The model under review builds one solid part; all positions refer to its coordinate system, in mm. Give positions to 0.01 mm unless a question says otherwise; leave off trailing zeros. Loops run counter-clockwise (first coordinate to the right, second up) from the corner with the lowest first, then second, coordinate; pieces in that order, holes last. Notation, with made-up numbers: M 22,-31 L 53,-31 A20 ccw 53,-21 Z; hole C 74,81.25 d3. An arc over 180 degrees is marked long. Return JSON: item names as keys, results as strings. Group by question number.
```python
from build123d import *
from build123d import SkipClean  # not in build123d's __all__

# Parameters (mm, degrees)
F1_DEPTH = 6


with BuildPart() as f1:
    # F0 (on Front) → F1 (new body)
    with BuildSketch(Plane.XZ):
        with BuildLine():
            ThreePointArc((-2.5981308411, 69.4027374984), (-23.7554424043, 60.1122052703), (-34.4088510941, 39.607310612))
            Line((-34.4088510941, 39.607310612), (-40, 0))
            Line((-40, 0), (0, 0))
            Line((0, 0), (0, 8))
            ThreePointArc((0, 8), (-26.7312756631, 33.7492995345), (-2, 61.4251288657))
            Line((-2, 61.4251288657), (-2.5981308411, 69.4027374984))
        make_face()
    extrude(amount=F1_DEPTH)

    # F2: F1 across plane


with BuildPart() as f1_1:
    add(f1.part, clean=False)
    with SkipClean():  # cleaning this boolean's faces spoils the solid; the shape is the same uncleaned
        add(f1.part.mirror(Plane.YZ), clean=False)


solid = f1_1.part
```
(1) Add section D-D (z = 7). Write out the cut boundary in (x, y).
(2) For pin 1 (1.5 mm diameter, centred on x = -4, y = -1.5, fed in from +Z); pin 2 (1.5 mm diameter, centred on x = 21.5, y = -1, fed in from +Z); pin 3 (1 mm diameter, centred on y = -4.5, z = 21.5, fed in from +X), all flat-tipped, find the tip position at first contact; note any pin that passes through.
(3) Add section A-A (x = -5.5). Write out the cut boundary in (y, z).
(4) For probe 1 along X at (y, z) = (-2, 15.5); probe 2 along Z at (x, y) = (21.5, -3.85); probe 3 along X at (y, z) = (-3.7, 58), list the stretches that pass through material, from the lowest coordinate up.
(5) Mouldability with a two-part tool opening along X and no side actions: class faces 1 (the flat face through (37.165, -2.958, 20.081)), 2 (the flat face through (2.3, -3, 65.4)), 3 (the flat face through (1, -3, 0)), 4 (the flat face through (-2.3, -3, 65.4)) as released by +X, released by -X, zero draft, split by the parting line, or undercut.
(6) Add section C-C (y = -5.15). Write out the cut boundary in (x, z).
(7) Add section B-B (z = 18). Write out the cut boundary in (x, y), and give its area (3 significant figures).
Verdict:
{
 "1": {"outline": "M -39.01,-6 L 39.01,-6 L 39.01,0 L -39.01,0 Z"},
 "2": {"pin 1": "stops at z = 69.35", "pin 2": "stops at z = 62.62", "pin 3": "stops at x = 37.04"},
 "3": {"outline": "M -6,0 L 0,0 L 0,8.57 L -6,8.57 Z; M -6,60.93 L 0,60.93 L 0,69.06 L -6,69.06 Z"},
 "4": {"probe 1": "x = -37.81 to -18.57, 18.57 to 37.81", "probe 2": "z = 0 to 18.83, 50.67 to 62.05", "probe 3": "x = -25.83 to -13.23, 13.23 to 25.83"},
 "5": {"face 1": "released by +X", "face 2": "undercut", "face 3": "zero draft", "face 4": "undercut"},
 "6": {"outline": "M -40,0 L 40,0 L 34.41,39.61 A34.75 ccw 2.6,69.4 L 2,61.43 A26.75 cw long -2,61.43 L -2.6,69.4 A34.75 ccw -34.41,39.61 Z"},
 "7": {"outline": "M -37.46,-6 L -20.86,-6 L -20.86,0 L -37.46,0 Z; M 20.86,-6 L 37.46,-6 L 37.46,0 L 20.86,0 Z", "area": "199 mm²"}
}
